Here's the drawing with two shaded views (mm, measured from the low corner). I have some questions. Round coordinates to 2 decimals unless told otherwise and drop trailing zeros. Order: outer loops, then holes, each group sorted by start corner. A loop starts at its lowest first (then second) coordinate and runs counter-clockwise, first axis right, second up. Notation, with made-up numbers: M 19.25,81 L 34.25,81 A34 cw 34.25,120 Z; hole C 70,65.5 d9. An arc over 180 degrees is marked long. One line per question, with ' | ' between items.
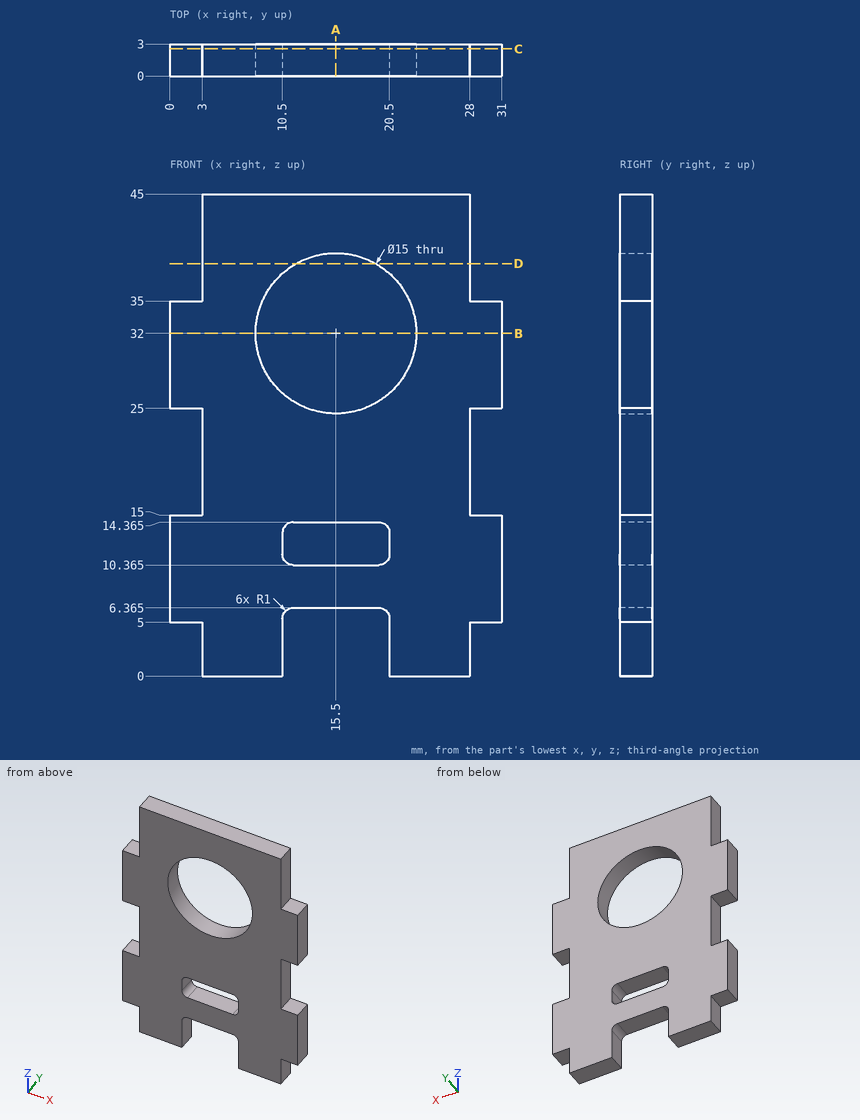
(1) Please list where these lines run through material, in increasing order: probe 1 along Z at (x, y) = (15.5, 1.55) (3 decimals); probe 2 along Z at (x, y) = (12, 0.25) (3 decimals); probe 3 along X at (y, z) = (2.4, 32). Write a range as [from, to].
Final values:
probe 1: [6.365, 10.365], [14.365, 24.5], [39.5, 45] | probe 2: [6.365, 10.365], [14.365, 25.367], [38.633, 45] | probe 3: [0, 8], [23, 31]
(2) If we section it at A-A on x = 15.5: Please give me the cut outline in (y, z) (3 decimals), plus the area to 3 significant figures.
Final values:
outline: M 0,6.365 L 3,6.365 L 3,10.365 L 0,10.365 Z; M 0,14.365 L 3,14.365 L 3,24.5 L 0,24.5 Z; M 0,39.5 L 3,39.5 L 3,45 L 0,45 Z | area: 58.9 mm^2
(3) If we section it at C-C on y = 2.55: State how many separate pieces and enclosed holes the cut face has, plus the area to 3 significant figures.
Final values:
separate pieces: 1 | enclosed holes: 2 | area: 966 mm^2
(4) If we section it at B-B on z = 32: Please give me the cut outline in (x, y).
Final values:
outline: M 0,0 L 8,0 L 8,3 L 0,3 Z; M 23,0 L 31,0 L 31,3 L 23,3 Z
(5) Will these pins go through, and if not, where does the flat tip stop? pin 1 Ø1.5 at (y, z) = (1.5, 21.5) entering from +X; pin 2 Ø0.9 at (x, y) = (15.5, 1.5) entering from -Z (3 decimals); pin 3 Ø0.9 at (y, z) = (1.5, 1.5) entering from -X.
Final values:
pin 1: x = 28 | pin 2: z = 6.365 | pin 3: x = 3
(6) If we section it at D-D on z = 38.5: Please give me the cut outline in (x, y).
Final values:
outline: M 3,0 L 11.76,0 L 11.76,3 L 3,3 Z; M 19.24,0 L 28,0 L 28,3 L 19.24,3 Z
